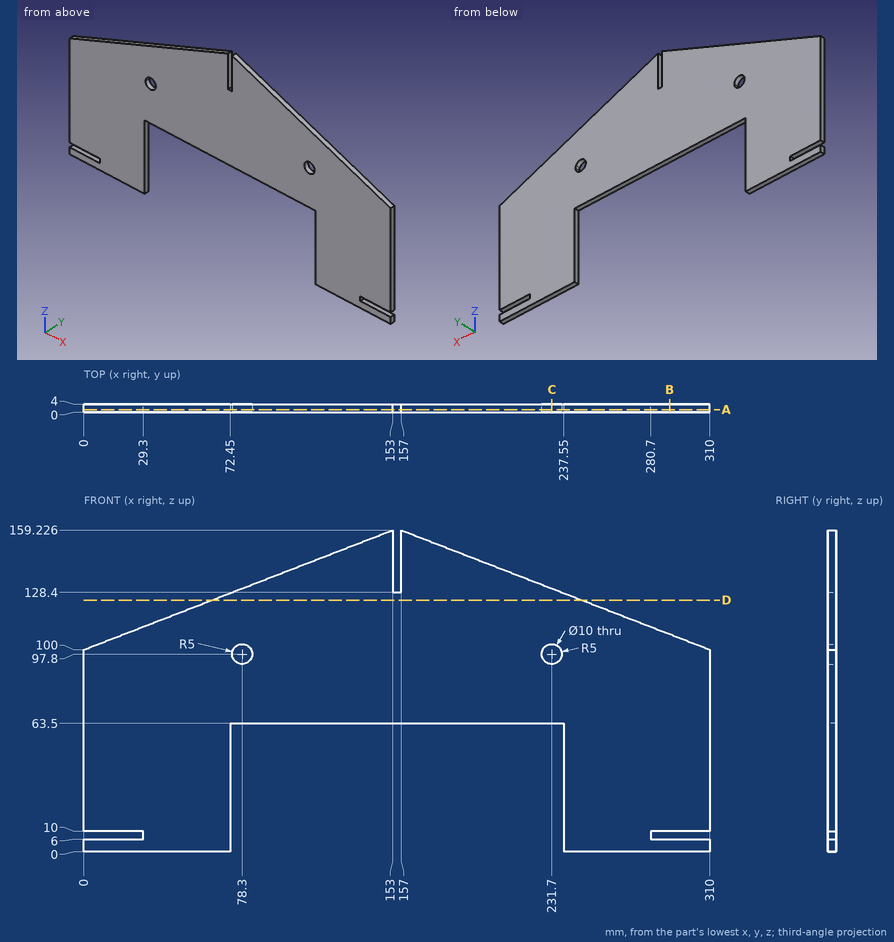
Source: three-view drawing plus pictorial views. Frame: mm from the lowest corner of the part. Coordinates: 2 decimals unless noted, no trailing zeros. Write each loop counter-clockwise with the first axis right and the second up, starting at its lowest first coordinate (ties: lowest second). Pieces come first, ordered by that corner, then holes. Notation, with made-up numbers: (34.5, 59.25) -> (81.5, 59.25) arc R29 cw to (81.5, 92.25) -> close; hole circle Ø1 at (6, 36.25). An arc over 180 degrees is marked (long way). Answer as a JSON object with one key per item and string values.
1. Section A-A on y = 1.2. Return the cut outline in (x, z), then the cut area to 3 significant figures.
Result set:
{"outline": "(0, 0) -> (72.45, 0) -> (72.45, 63.5) -> (237.55, 63.5) -> (237.55, 0) -> (310, 0) -> (310, 6) -> (280.7, 6) -> (280.7, 10) -> (310, 10) -> (310, 100) -> (157, 159.23) -> (157, 128.4) -> (153, 128.4) -> (153, 159.23) -> (0, 100) -> (0, 10) -> (29.3, 10) -> (29.3, 6) -> (0, 6) -> close; hole circle Ø10 at (78.3, 97.8); hole circle Ø10 at (231.7, 97.8)", "area": "29,300 mm2"}
2. Section B-B on x = 290. Return the cut outline in (y, z).
Result set:
{"outline": "(0, 0) -> (4, 0) -> (4, 6) -> (0, 6) -> close; (0, 10) -> (4, 10) -> (4, 107.74) -> (0, 107.74) -> close"}
3. Material intervals for line 1 (X direction, y = 1.4, z = 97.8); line 2 (X direction, y = 2.45, z = 10.5); line 3 (X direction, y = 2, z = 96) (1 decimal), sorted ascending. Write a range as from..to.
Result set:
{"line 1": "x = 0..73.3, 83.3..226.7, 236.7..310", "line 2": "x = 0..72.45, 237.55..310", "line 3": "x = 0..73.6, 83..227, 236.4..310"}
4. First-contact query: P1, Ø2, axis at x = 155.5, y = 1, coming from the +Z side; P2, Ø8, axis at x = 120, z = 116.5, coming from the -Y side; P3, Ø1.5, axis at x = 108, y = 2, coming from the +Z side; P4, Ø9, axis at x = 231.7, z = 97.8, coming from the -Y side. Flat tips, straight axial feed; report the tip coordinate or a pass-through.
Result set:
{"P1": "stops at z = 128.4", "P2": "stops at y = 0", "P3": "stops at z = 142.1", "P4": "passes through"}
5. Section C-C on x = 231.7. Return the cut outline in (y, z), then the cut area to 3 significant figures.
Result set:
{"outline": "(0, 63.5) -> (4, 63.5) -> (4, 92.8) -> (0, 92.8) -> close; (0, 102.8) -> (4, 102.8) -> (4, 130.31) -> (0, 130.31) -> close", "area": "227 mm2"}
6. Section D-D on z = 124.5. Return the cut outline in (x, y).
Result set:
{"outline": "(63.29, 0) -> (246.71, 0) -> (246.71, 4) -> (63.29, 4) -> close"}
